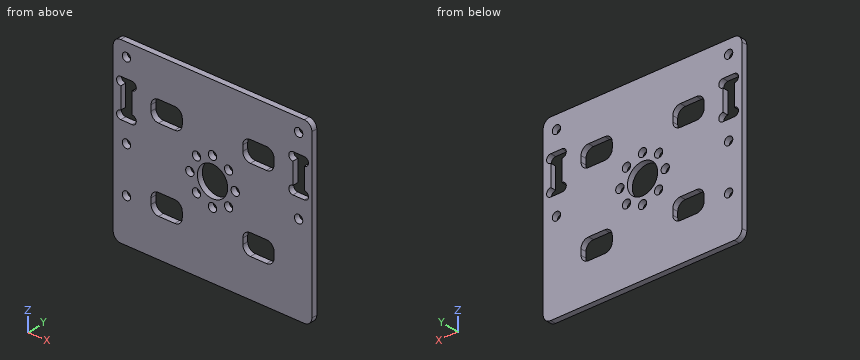
Autodesk Inventor part; units mm, degrees
ref_plane "YZ Plane" through (0, 0, 0) normal (1, 0, 0) x (0, 1, 0)
ref_plane "XZ Plane" through (0, 0, 0) normal (0, 1, 0) x (-1, 0, 0)
ref_plane "XY Plane" through (0, 0, 0) normal (0, 0, 1) x (1, 0, 0)
sketch "スケッチ1" plane through (0, 0, 0) normal (0, 1, 0) x (-1, 0, 0)
  circle A0 centre (0, 0) radius 4
  circle A1 centre (0, 0) radius 8
  circle A2 centre (0, 0) radius 6 construction
  circle A3 centre (0, -6) radius 1.1
  circle A4 centre (4.2426, -4.2426) radius 1.1
  circle A5 centre (6, 0) radius 1.1
  circle A6 centre (4.2426, 4.2426) radius 1.1
  circle A7 centre (0, 6) radius 1.1
  circle A8 centre (-4.2426, 4.2426) radius 1.1
  circle A9 centre (-6, 0) radius 1.1
  circle A10 centre (-4.2426, -4.2426) radius 1.1
  line L0 (26.25, -23.5) -> (-26.25, -23.5)
  line L1 (-26.25, -23.5) -> (-26.25, 23.5)
  line L2 (-26.25, 23.5) -> (26.25, 23.5)
  line L3 (26.25, 23.5) -> (26.25, -23.5)
  line L4 (26.25, -23.5) -> (-26.25, 23.5) construction
  line L5 (-26.25, -23.5) -> (26.25, 23.5) construction
  line L6 (24.25, 5) -> (21.25, 5)
  line L7 (21.25, 5) -> (21.25, 15)
  line L8 (21.25, 15) -> (24.25, 15)
  line L9 (24.25, 15) -> (24.25, 5)
  circle A11 centre (24.25, 6.1) radius 1.1
  circle A12 centre (21.25, 6.1) radius 1.1
  line L10 (0, 0) -> (0, -23.5) construction
  circle A13 centre (24.25, 13.9) radius 1.1
  circle A14 centre (21.25, 13.9) radius 1.1
  line L11 (-24.25, 5) -> (-21.25, 5)
  line L12 (-21.25, 5) -> (-21.25, 15)
  line L13 (-21.25, 15) -> (-24.25, 15)
  line L14 (-24.25, 15) -> (-24.25, 5)
  circle A15 centre (-24.25, 6.1) radius 1.1
  circle A16 centre (-21.25, 6.1) radius 1.1
  circle A17 centre (-24.25, 13.9) radius 1.1
  circle A18 centre (-21.25, 13.9) radius 1.1
  circle A19 centre (22.75, 0) radius 1.1
  circle A20 centre (22.75, 20) radius 1.1
  circle A21 centre (-22.75, 0) radius 1.1
  circle A22 centre (-22.75, 20) radius 1.1
  circle A23 centre (22.75, 20) radius 3.5 construction
  point P0 (21.25, 10)
  point P1 (-21.25, 10)
  point P2 (22.75, 5)
  point P3 (-21.25, 12.8)
  point P4 (-21.25, 7.2)
  point P5 (-24.25, 7.2)
  point P6 (-24.25, 12.8)
  point P7 (-24.25, 15)
  point P8 (21.25, 12.8)
  point P9 (21.25, 15)
  point P10 (24.25, 15)
  point P11 (24.25, 12.8)
  point P12 (24.25, 7.2)
  point P13 (21.25, 7.2)
  point P14 (22.75, 15)
  dimension "d2" = 12
  dimension "d10" = 2.2
  dimension "d0" = 8
  dimension "d1" = 16
  dimension "d3" = 2.2
  dimension "d6" = 360
  dimension "d8" = 3
  dimension "d9" = 10
  dimension "d11" = 42.5
  dimension "d12" = 2.2
  dimension "d13" = 5
  dimension "d17" = 5
  dimension "d18" = 7
extrude "押し出し1" add sketch "スケッチ1" along normal blind 1.5 contours A1 | L0 L1 L2 L3
sketch "スケッチ2" plane through (0, 0, 0) normal (0, -1, 0) x (1, 0, 0)
  circle A0 centre (-22.75, -12) radius 1.1
  circle A1 centre (-22.75, 0) radius 1.1
  point P0 (0, 0)
  dimension "d19" = 2.2
  dimension "d20" = 12
extrude "押し出し2" cut sketch "スケッチ2" against normal through all contours A0
fillet "フィレット1" radius 2 4 edges at (-26.25, 0.75, -23.5) (26.25, 0.75, -23.5) (26.25, 0.75, 23.5) (-26.25, 0.75, 23.5)
sketch "スケッチ3" plane through (0, 1.5, 0) normal (0, 1, 0) x (1, 0, 0)
  arc A0 (-26.25, -21.5) -> (-24.25, -23.5) centre (-24.25, -21.5) ccw
  line L0 (-24.25, -23.5) -> (24.25, -23.5)
  arc A1 (24.25, -23.5) -> (26.25, -21.5) centre (24.25, -21.5) ccw
  line L1 (26.25, -21.5) -> (26.25, 21.5)
  arc A2 (26.25, 21.5) -> (24.25, 23.5) centre (24.25, 21.5) ccw
  line L2 (24.25, 23.5) -> (-24.25, 23.5)
  arc A3 (-24.25, 23.5) -> (-26.25, 21.5) centre (-24.25, 21.5) ccw
  line L3 (-26.25, 21.5) -> (-26.25, -21.5)
  circle A4 centre (-22.75, 12) radius 1.1
  circle A5 centre (22.75, -20) radius 1.1
  circle A6 centre (-22.75, -20) radius 1.1
  circle A7 centre (-22.75, 0) radius 1.1
  line L4 (21.25, -12.8) -> (21.25, -7.2)
  arc A8 (21.25, -5) -> (21.25, -7.2) centre (21.25, -6.1) ccw
  line L5 (21.25, -5) -> (24.25, -5)
  arc A9 (24.25, -7.2) -> (24.25, -5) centre (24.25, -6.1) ccw
  line L6 (24.25, -7.2) -> (24.25, -12.8)
  arc A10 (24.25, -15) -> (24.25, -12.8) centre (24.25, -13.9) ccw
  line L7 (24.25, -15) -> (21.25, -15)
  arc A11 (21.25, -12.8) -> (21.25, -15) centre (21.25, -13.9) ccw
  arc A12 (-21.25, -15) -> (-21.25, -12.8) centre (-21.25, -13.9) ccw
  line L8 (-21.25, -15) -> (-24.25, -15)
  arc A13 (-24.25, -12.8) -> (-24.25, -15) centre (-24.25, -13.9) ccw
  line L9 (-24.25, -12.8) -> (-24.25, -7.2)
  arc A14 (-24.25, -5) -> (-24.25, -7.2) centre (-24.25, -6.1) ccw
  line L10 (-24.25, -5) -> (-21.25, -5)
  arc A15 (-21.25, -7.2) -> (-21.25, -5) centre (-21.25, -6.1) ccw
  line L11 (-21.25, -7.2) -> (-21.25, -12.8)
  circle A16 centre (6, 0) radius 1.1
  circle A17 centre (0, -6) radius 1.1
  circle A18 centre (-6, 0) radius 1.1
  circle A19 centre (0, 6) radius 1.1
  circle A20 centre (22.75, 0) radius 1.1
  circle A21 centre (4.2426, 4.2426) radius 1.1
  circle A22 centre (4.2426, -4.2426) radius 1.1
  circle A23 centre (-4.2426, -4.2426) radius 1.1
  circle A24 centre (-4.2426, 4.2426) radius 1.1
  circle A25 centre (0, 0) radius 4
  circle A26 centre (0, 0) radius 8
  line L12 (-16.25, -13.5) -> (16.25, -13.5)
  line L13 (16.25, -13.5) -> (16.25, 13.5)
  line L14 (16.25, 13.5) -> (-16.25, 13.5)
  line L15 (-16.25, 13.5) -> (-16.25, -13.5)
  line L16 (-8, 0) -> (-8, -13.5)
  line L17 (8, 0) -> (8, -13.5)
  line L18 (-8, 0) -> (-8, 13.5)
  line L19 (8, 0) -> (8, 13.5)
  line L20 (0, -8) -> (-16.25, -8)
  line L21 (-16.25, 8) -> (0, 8)
  line L22 (0, 8) -> (16.25, 8)
  line L23 (0, -8) -> (16.25, -8)
  point P0 (-8, 8)
  point P1 (8, 8)
  point P2 (8, -8)
  point P3 (-8, -8)
  dimension "d24" = 16
  dimension "d25" = 10
extrude "押し出し3" cut sketch "スケッチ3" against normal through all contours L23 L13 L12 L17 | L19 L14 L13 L22 | L21 L15 L14 L18 | L16 L12 L15 L20
fillet "フィレット2" radius 2 16 edges at (-16.25, 0.75, 8) (-16.25, 0.75, 13.5) (-8, 0.75, 13.5) (-8, 0.75, 8) (8, 0.75, 13.5) (16.25, 0.75, 13.5) (16.25, 0.75, 8) (8, 0.75, 8) (16.25, 0.75, -8) (16.25, 0.75, -13.5) (8, 0.75, -13.5) (8, 0.75, -8) (-8, 0.75, -8) (-16.25, 0.75, -13.5) (-16.25, 0.75, -8) (-8, 0.75, -13.5)
properties part number "kosi_v3_1.5" material "アルミニウム 2014-T4"
Input: part model. Units: mm. Frame: model coordinates. Give positions to 0.01 mm unless a question says otherwise; leave off trailing zeros. Loops run counter-clockwise (first coordinate to the right, second up) from the corner with the lowest first, then second, coordinate; pieces in that order, holes last. Notation, with made-up numbers: (-28, 79.25) - (-19, 79.25) arc R21 cw to (-19, 115.25) - close; hole circle Ø1 at (-14.5, 66.5). An arc over 180 degrees is marked (long way). Use CSV: the item, a comma, the result in double quotes. Start each with the question number.
Item 1: Line query: line 1 (Z direction, x = 0, y = 0.4); line 2 (Z direction, x = 4.5, y = 1.3); line 3 (Z direction, x = -8.5, y = 0.1). Output: solid intervals per line, ascending.
Item 2: Section A-A on z = 20. Return loops of the section in (x, y).
Item 3: Section B-B on x = 22.75. Return loops of the section in (y, z).
Item 4: Section C-C on z = -6. Return loops of the section in (x, y).
Item 5: Section D-D on x = 6. Return loops of the section in (y, z).
Ans:
1,line 1,"z = -23.5 to -7.1, -4.9 to -4, 4 to 4.9, 7.1 to 23.5"
1,line 2,"z = -23.5 to -5.31, -3.17 to 3.17, 5.31 to 23.5"
1,line 3,"z = -23.5 to -12.82, -8.68 to 8.68, 12.82 to 23.5"
2,outline,"(-26.25, 0) - (-23.85, 0) - (-23.85, 1.5) - (-26.25, 1.5) - close; (-21.65, 0) - (21.65, 0) - (21.65, 1.5) - (-21.65, 1.5) - close; (23.85, 0) - (26.25, 0) - (26.25, 1.5) - (23.85, 1.5) - close"
3,outline,"(0, -23.5) - (1.5, -23.5) - (1.5, -1.1) - (0, -1.1) - close; (0, 1.1) - (1.5, 1.1) - (1.5, 5) - (0, 5) - close; (0, 15) - (1.5, 15) - (1.5, 18.9) - (0, 18.9) - close; (0, 21.1) - (1.5, 21.1) - (1.5, 23.5) - (0, 23.5) - close"
4,outline,"(-26.25, 0) - (-1.1, 0) - (-1.1, 1.5) - (-26.25, 1.5) - close; (1.1, 0) - (26.25, 0) - (26.25, 1.5) - (1.1, 1.5) - close"
5,outline,"(0, -23.5) - (1.5, -23.5) - (1.5, -1.1) - (0, -1.1) - close; (0, 1.1) - (1.5, 1.1) - (1.5, 23.5) - (0, 23.5) - close"
